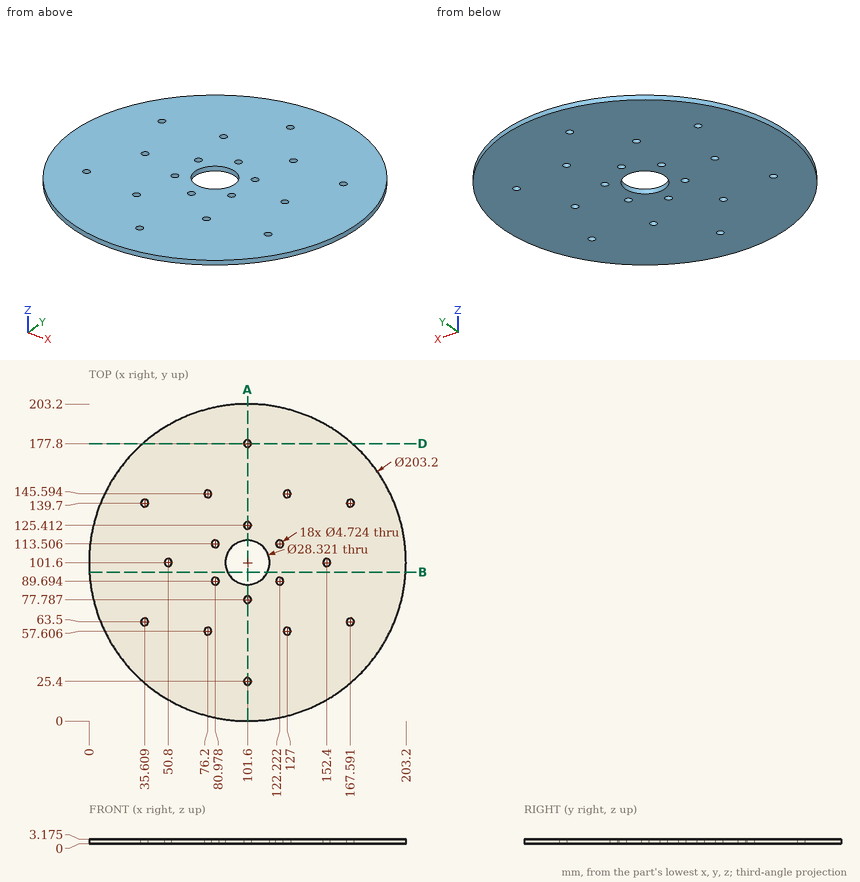
Check sheet for the drawn part. Datum: minimum x, y, z corner. Units: mm. Coordinates: 2 decimals unless noted, no trailing zeros. Loops run counter-clockwise (first coordinate to the right, second up) from the corner with the lowest first, then second, coordinate; pieces in that order, holes last. Notation, with made-up numbers: (34, 38.25) -> (85, 38.25) arc R12 cw to (85, 59.25) -> close; hole circle Ø5 at (85, 86). An arc over 180 degrees is marked (long way). Write each question's results on one line, items separated by ' | '.
Item 1: Material ranges on L1, parallel to X at y = 139.7, z = 2 (1 decimal); L2, parallel to Y at x = 35, z = 2.7 (1 decimal); L3, parallel to Y at x = 81, z = 1.2 (1 decimal), recorded low to high.
Found:
L1: x = 7.4 to 33.2, 38 to 165.2, 170 to 195.8 | L2: y = 24.9 to 61.2, 65.8 to 137.4, 142 to 178.3 | L3: y = 2.1 to 87.3, 92.1 to 111.1, 115.9 to 201.1
Item 2: Section check D-D, the plane y = 177.8. Enter the section's corners in (x, z) (1 decimal).
Found:
outline: (34.4, 0) -> (99.2, 0) -> (99.2, 3.2) -> (34.4, 3.2) -> close; (104, 0) -> (168.8, 0) -> (168.8, 3.2) -> (104, 3.2) -> close
Item 3: Gauge pin test, flat end, axial feed: pin 1 (7.5 mm diameter, centred on x = 167.59, y = 63.5, fed in from +Z) (1 decimal). Record the tip position at first contact, or that the pin passes through.
Found:
pin 1: stops at z = 3.2
Item 4: Section check A-A, the plane x = 101.6. Count the separate pieces of the cut face and the enclosed holes in it.
Found:
separate pieces: 6 | enclosed holes: 0
Item 5: Section check B-B, the plane y = 95.5. Enter the section's corners in (x, z) (1 decimal).
Found:
outline: (0.2, 0) -> (88.8, 0) -> (88.8, 3.2) -> (0.2, 3.2) -> close; (114.4, 0) -> (203, 0) -> (203, 3.2) -> (114.4, 3.2) -> close
